Check sheet for the modelled part. Datum: model origin and axes. Units: mm. Round coordinates to 2 decimals unless told otherwise and drop trailing zeros. Order: outer loops, then holes, each group sorted by start corner. A loop starts at its lowest first (then second) coordinate and runs counter-clockwise, first axis right, second up. Notation, with made-up numbers: M 27.5,86.25 L 85.5,86.25 A18 cw 85.5,100.25 Z; hole C 63,39.5 d9. An arc over 180 degrees is marked long. One line per item, written item: value. Start each with the question number.
(1) Cross-section at C-C, the plane z = -0.7. Count the separate pieces of the cut face and the enclosed holes in it, and give its area (3 significant figures).
(2) Release check for a two-part mould opening along Y. For faces 1 (the face through (-2, 0, 0)), 2 (the face through (50.12, 42, 0)), 3 (the face through (-77.925, 42, 0)) record: released by +Y, released by -Y, zero draft, split by the parting line, or undercut.
(3) Depth check by flat-ended pin: pin 1 Ø0.9 at (y, z) = (42.5, 0) entering from +X; pin 2 Ø3 at (x, y) = (-67.93, 48.2) entering from +Z. Enter the tip coordinate at first touch or a pass-through.
(4) Thickness scan on L1, parallel to X at y = 58, z = -0.55; L2, parallel to Y at x = -1, z = -1.2; L3, parallel to X at y = 78, z = 0.3. Record the ranges inside material, lowest first.
(5) Cross-section at D-D, the plane y = 8. Enter the section's corners in (x, z).
(6) Cross-section at A-A, the plane y = 23. Enter the section's corners in (x, z), and give its area (3 significant figures).
(7) Cross-section at B-B, the plane x = -1. Enter the section's corners in (y, z).
from build123d import *

# Parameters (mm, degrees)
ESQUISSE2_W             = 154.98
ESQUISSE2_H             = 3
BOSS_EXTRU_1_DEPTH      = 64.27
ESQUISSE3_R             = 2.5
ENL_V_MAT_EXTRU_1_DEPTH = 102.054178938
ENL_V_MAT_EXTRU_2_DEPTH = 102.054178938
SKETCH1_W               = 155.004364221
SKETCH1_H               = 20
BOSS_EXTRUDE1_DEPTH     = 3
CUT_EXTRUDE1_DEPTH      = 10


with BuildPart() as part:
    # Esquisse2 → Boss.-Extru.1 (new body)
    with BuildSketch(Plane(origin=(0, 0, 0), x_dir=(1, 0, 0), z_dir=(0, 1, 0))):
        with Locations((-0.435054897, 0)):
            Rectangle(ESQUISSE2_W, ESQUISSE2_H)
    extrude(amount=BOSS_EXTRU_1_DEPTH)

    # Esquisse3 → Enlèv. mat.-Extru.1 (cut, through all)
    with BuildSketch(Plane.XY.offset(1.5)):
        with Locations((-67.925054897, 16.0675)):
            Circle(ESQUISSE3_R)
        with Locations((-67.925054897, 48.2025)):
            Circle(ESQUISSE3_R)
        with Locations((67.054945103, 48.2025)):
            Circle(ESQUISSE3_R)
        with Locations((67.054945103, 16.0675)):
            Circle(ESQUISSE3_R)
    extrude(amount=-ENL_V_MAT_EXTRU_1_DEPTH, mode=Mode.SUBTRACT)

    # Esquisse4 → Enlèv. mat.-Extru.2 (cut, through all)
    with BuildSketch(Plane.XY.offset(1.5)):
        with BuildLine():
            Line((-41.680054897, 47.135), (-41.680054897, 17.135))
            ThreePointArc((-41.680054897, 17.135), (-39.180054897, 14.635), (-36.680054897, 17.135))
            Line((-36.680054897, 17.135), (-36.680054897, 47.135))
            ThreePointArc((-36.680054897, 47.135), (-39.180054897, 49.635), (-41.680054897, 47.135))
        make_face()
        with BuildLine():
            Line((-2.935054897, 47.135), (-2.935054897, 17.135))
            ThreePointArc((-2.935054897, 17.135), (-0.435054897, 14.635), (2.064945103, 17.135))
            Line((2.064945103, 17.135), (2.064945103, 47.135))
            ThreePointArc((2.064945103, 47.135), (-0.435054897, 49.635), (-2.935054897, 47.135))
        make_face()
        with BuildLine():
            Line((35.809945103, 47.135), (35.809945103, 17.135))
            ThreePointArc((35.809945103, 17.135), (38.309945103, 14.635), (40.809945103, 17.135))
            Line((40.809945103, 17.135), (40.809945103, 47.135))
            ThreePointArc((40.809945103, 47.135), (38.309945103, 49.635), (35.809945103, 47.135))
        make_face()
    extrude(amount=-ENL_V_MAT_EXTRU_2_DEPTH, mode=Mode.SUBTRACT)

    # Sketch1 → Boss-Extrude1 (add)
    with BuildSketch(Plane.XY.offset(1.5)):
        with Locations((-0.422872787, 74.27)):
            Rectangle(SKETCH1_W, SKETCH1_H)
    extrude(amount=-BOSS_EXTRUDE1_DEPTH)

    # Sketch2 → Cut-Extrude1 (cut)
    with BuildSketch(Plane.XY.offset(1.5)):
        with BuildLine():
            Line((-27.180054897, 67.135), (-27.180054897, 17.135))
            ThreePointArc((-27.180054897, 17.135), (-39.180054897, 5.135), (-51.180054897, 17.135))
            Line((-51.180054897, 17.135), (-51.180054897, 67.135))
            ThreePointArc((-51.180054897, 67.135), (-39.180054897, 79.135), (-27.180054897, 67.135))
        make_face()
        with BuildLine():
            Line((-12.530054897, 67.135), (-12.530054897, 17.135))
            ThreePointArc((-12.530054897, 17.135), (-0.530054897, 5.135), (11.469945103, 17.135))
            Line((11.469945103, 17.135), (11.469945103, 67.135))
            ThreePointArc((11.469945103, 67.135), (-0.530054897, 79.135), (-12.530054897, 67.135))
        make_face()
        with BuildLine():
            Line((26.119945103, 67.135), (26.119945103, 17.135))
            ThreePointArc((26.119945103, 17.135), (38.119945103, 5.135), (50.119945103, 17.135))
            Line((50.119945103, 17.135), (50.119945103, 67.135))
            ThreePointArc((50.119945103, 67.135), (38.119945103, 79.135), (26.119945103, 67.135))
        make_face()
    extrude(amount=-CUT_EXTRUDE1_DEPTH, mode=Mode.SUBTRACT)


solid = part.part
Values found:
1. separate pieces: 1
1. enclosed holes: 7
1. area: 8,020 mm^2
2. face 1: released by -Y
2. face 2: undercut
2. face 3: zero draft
3. pin 1: x = 77.05
3. pin 2: through
4. L1: -77.93 to -51.18, -27.18 to -12.53, 11.47 to 26.12, 50.12 to 77.05
4. L2: 0 to 5.14, 79.13 to 84.27
4. L3: -77.93 to -44.27, -34.09 to -5.62, 4.56 to 33.03, 43.21 to 77.08
5. outline: M -77.93,-1.5 L -46.96,-1.5 L -46.96,1.5 L -77.93,1.5 Z; M -31.4,-1.5 L -8.31,-1.5 L -8.31,1.5 L -31.4,1.5 Z; M 7.25,-1.5 L 30.34,-1.5 L 30.34,1.5 L 7.25,1.5 Z; M 45.9,-1.5 L 77.05,-1.5 L 77.05,1.5 L 45.9,1.5 Z
6. outline: M -77.93,-1.5 L -51.18,-1.5 L -51.18,1.5 L -77.93,1.5 Z; M -27.18,-1.5 L -12.53,-1.5 L -12.53,1.5 L -27.18,1.5 Z; M 11.47,-1.5 L 26.12,-1.5 L 26.12,1.5 L 11.47,1.5 Z; M 50.12,-1.5 L 77.05,-1.5 L 77.05,1.5 L 50.12,1.5 Z
6. area: 249 mm^2
7. outline: M 0,-1.5 L 5.14,-1.5 L 5.14,1.5 L 0,1.5 Z; M 79.13,-1.5 L 84.27,-1.5 L 84.27,1.5 L 79.13,1.5 Z
